```python
from build123d import *

# Parameters (mm, degrees)
BOSS_EXTRUDE1_DEPTH = 17.4625
VARFILLET1_START    = -17.4625
VARFILLET1_DEPTH    = 34.925
VARFILLET1_START_2  = -18
VARFILLET1_2_DEPTH  = 36
VARFILLET1_START_3  = -11
VARFILLET1_3_DEPTH  = 6
CUT_EXTRUDE1_DEPTH  = 34.925


with BuildPart() as part:
    # Sketch1 → Boss-Extrude1 (new, symmetric)
    with BuildSketch(Plane.XY):
        with BuildLine():
            Line((-13.335, 0), (-13.335, -6.35))
            Line((-13.335, -6.35), (-43.4975, -6.35))
            Line((-43.4975, -6.35), (-43.4975, -9.525))
            Line((-43.4975, -9.525), (-10.16, -9.525))
            Line((-10.16, -9.525), (-10.16, 0))
            ThreePointArc((-10.16, 0), (3e-07, 10.16), (10.16, -6e-07))
            Line((10.16, -6e-07), (10.16, -9.525))
            Line((10.16, -9.525), (43.4975, -9.525))
            Line((43.4975, -9.525), (43.4975, -6.35))
            Line((43.4975, -6.35), (13.335, -6.35))
            Line((13.335, -6.35), (13.335, 0))
            ThreePointArc((13.335, 0), (0, 13.335), (-13.335, 0))
        make_face()
    extrude(amount=BOSS_EXTRUDE1_DEPTH, both=True)

    # VarFillet1: read off the stored shape, not the designer's step
    # VarFillet1 outline → VarFillet1 (add)
    with BuildSketch(Plane.XY.offset(VARFILLET1_START)):
        with BuildLine():
            add(Edge.make_bspline(
                [(13.335, -3.81), (13.335, -6.35), (15.875, -6.35)],
                knots=[0, 0, 0, 1, 1, 1], degree=2, weights=[1, 0.707106781, 1]))
            Line((13.335, -3.81), (13.335, -6.35))
            Line((13.335, -6.35), (15.875, -6.35))
        make_face()
        with BuildLine():
            add(Edge.make_bspline(
                [(-15.875, -6.35), (-13.335, -6.35), (-13.335, -3.81)],
                knots=[0, 0, 0, 1, 1, 1], degree=2, weights=[1, 0.707106781, 1]))
            Line((-15.875, -6.35), (-13.335, -6.35))
            Line((-13.335, -6.35), (-13.335, -3.81))
        make_face()
    extrude(amount=VARFILLET1_DEPTH)

    # VarFillet1 2 outline → VarFillet1 2 (cut)
    with BuildSketch(Plane.XY.offset(VARFILLET1_START_2)):
        with BuildLine():
            Line((10.16, -9.525), (12.7, -9.525))
            add(Edge.make_bspline(
                [(12.7, -9.525), (10.16, -9.525), (10.16, -6.985)],
                knots=[0, 0, 0, 1, 1, 1], degree=2, weights=[1, 0.707106781, 1]))
            Line((10.16, -6.985), (10.16, -9.525))
        make_face()
        with BuildLine():
            Line((-10.16, -9.525), (-10.16, -6.985))
            add(Edge.make_bspline(
                [(-10.16, -6.985), (-10.16, -9.525), (-12.7, -9.525)],
                knots=[0, 0, 0, 1, 1, 1], degree=2, weights=[1, 0.707106781, 1]))
            Line((-12.7, -9.525), (-10.16, -9.525))
        make_face()
    extrude(amount=VARFILLET1_2_DEPTH, mode=Mode.SUBTRACT)

    # VarFillet1 3 outline → VarFillet1 3 (cut)
    with BuildSketch(Plane(origin=(0, 0, 0), x_dir=(1, 0, 0), z_dir=(0, 1, 0)).offset(VARFILLET1_START_3)):
        with BuildLine():
            Line((-43.4975, 17.4625), (-43.4975, 14.9225))
            add(Edge.make_bspline(
                [(-43.4975, 14.9225), (-43.4975, 17.4625), (-40.9575, 17.4625)],
                knots=[0, 0, 0, 1, 1, 1], degree=2, weights=[1, 0.707106781, 1]))
            Line((-40.9575, 17.4625), (-43.4975, 17.4625))
        make_face()
        with BuildLine():
            add(Edge.make_bspline(
                [(-40.9575, -17.4625), (-43.4975, -17.4625), (-43.4975, -14.9225)],
                knots=[0, 0, 0, 1, 1, 1], degree=2, weights=[1, 0.707106781, 1]))
            Line((-43.4975, -14.9225), (-43.4975, -17.4625))
            Line((-43.4975, -17.4625), (-40.9575, -17.4625))
        make_face()
        with BuildLine():
            Line((43.4975, 17.4625), (40.9575, 17.4625))
            add(Edge.make_bspline(
                [(43.4975, 14.9225), (43.4975, 17.4625), (40.9575, 17.4625)],
                knots=[0, 0, 0, 1, 1, 1], degree=2, weights=[1, 0.707106781, 1]))
            Line((43.4975, 14.9225), (43.4975, 17.4625))
        make_face()
        with BuildLine():
            add(Edge.make_bspline(
                [(40.9575, -17.4625), (43.4975, -17.4625), (43.4975, -14.9225)],
                knots=[0, 0, 0, 1, 1, 1], degree=2, weights=[1, 0.707106781, 1]))
            Line((40.9575, -17.4625), (43.4975, -17.4625))
            Line((43.4975, -17.4625), (43.4975, -14.9225))
        make_face()
    extrude(amount=VARFILLET1_3_DEPTH, mode=Mode.SUBTRACT)

    # Sketch2 → Cut-Extrude1 (cut)
    with BuildSketch(Plane(origin=(0, 0, 0), x_dir=(1, 0, 0), z_dir=(0, 1, 0))):
        with BuildLine():
            Line((-34.76625, 3.96875), (-26.82875, 3.96875))
            ThreePointArc((-26.82875, 3.96875), (-22.86, 0), (-26.82875, -3.96875))
            Line((-26.82875, -3.96875), (-34.76625, -3.96875))
            ThreePointArc((-34.76625, -3.96875), (-38.735, 0), (-34.76625, 3.96875))
        make_face()
        with BuildLine():
            Line((34.76625, -3.96875), (26.82875, -3.96875))
            ThreePointArc((26.82875, -3.96875), (22.86, 0), (26.82875, 3.96875))
            Line((26.82875, 3.96875), (34.76625, 3.96875))
            ThreePointArc((34.76625, 3.96875), (38.735, 0), (34.76625, -3.96875))
        make_face()
    extrude(amount=-CUT_EXTRUDE1_DEPTH, mode=Mode.SUBTRACT)


solid = part.part
```
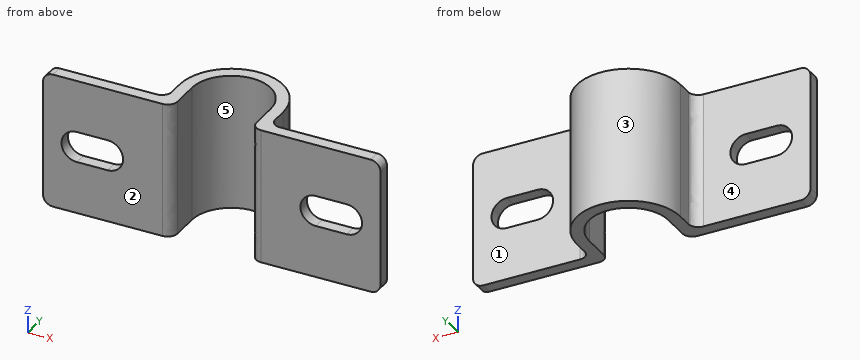
Build history of the part. All positions in model axes, mm. Face numbers are marked on the shaded views. A direction names the side the tool comes from. Give positions to 0.01 mm unless a question says otherwise; leave off trailing zeros. Order: outer loops, then holes, each group sorted by start corner. A loop starts at its lowest first (then second) coordinate and runs counter-clockwise, first axis right, second up. Notation, with made-up numbers: M 73.5,89.25 L 125.5,89.25 A26 ccw 125.5,103.25 Z; hole C 72,14.25 d1. An arc over 180 degrees is marked long. Return JSON: item names as keys, results as strings.
Q1. Flat gauge pins, fed straight in: pin 1 (6 mm diameter, centred on y = -0.5, z = -13.5, fed in from +X) (3 decimals); pin 2 (3.5 mm diameter, centred on y = -3.5, z = 0, fed in from -X); pin 3 (12 mm diameter, centred on y = 8.5, z = -7, fed in from +X). Where does each tip first touch, or does it go through?
Answer list:
{"pin 1": "stops at x = 13.335", "pin 2": "stops at x = -13.78", "pin 3": "stops at x = 13.1"}
Q2. Band-saw the part on D-D (x = 0). Give the cut face in (y, z) (1 decimal).
Answer list:
{"outline": "M 10.2,-17.5 L 13.3,-17.5 L 13.3,17.5 L 10.2,17.5 Z"}
Q3. 3-axis set-ups, long thin cutter, end or side, ignore diameter. For the marked faces 1 and 2: which of +Z, -Z, +X, -X, +Y, -Y reach the whole face in a straight line?
Answer list:
{"face 1": "+Z, -Z, +X, +Y", "face 2": "+Z, -Z, +X, -X, -Y"}
Q4. Two-plate mould, pull along X, no slides. Class the marked faces 3, 4 and 5: pulls with the +X half, pulls with the -X half, needs draft (parallel to the pull), parting line crosses it, or undercut.
Answer list:
{"face 3": "parting line crosses it", "face 4": "needs draft", "face 5": "undercut"}
Q5. Band-saw the part on C-C (z = 0). Count the separate pieces of the cut face and the enclosed holes in it, then the cut area to 3 significant figures.
Answer list:
{"separate pieces": "3", "enclosed holes": "0", "area": "268 mm^2"}
Q6. Wall check: probe 1 along X at (y, z) = (-2.5, 4) (3 decimals); probe 2 along Y at (x, z) = (21, -9) (3 decimals); probe 3 along Z at (x, y) = (-28, -7.25). Give the ranges that are in metal, low to high. Write a range as from..to.
Answer list:
{"probe 1": "x = -13.335..-10.16, 10.16..13.335", "probe 2": "y = -9.525..-6.35", "probe 3": "z = -17.46..-3.97, 3.97..17.46"}
Q7. Band-saw the part on B-B (y = -2.75). Give the cut face in (x, z) (1 decimal), then the cut area to 3 significant figures.
Answer list:
{"outline": "M -13.3,-17.5 L -10.2,-17.5 L -10.2,17.5 L -13.3,17.5 Z; M 10.2,-17.5 L 13.3,-17.5 L 13.3,17.5 L 10.2,17.5 Z", "area": "222 mm^2"}
